CAD build for the part. Positions are in the model's coordinates, mm. Give positions to 0.01 mm unless a question says otherwise; leave off trailing zeros. Write each loop counter-clockwise with the first axis right and the second up, starting at its lowest first coordinate (ties: lowest second). Pieces come first, ordered by that corner, then holes. Notation, with made-up numbers: (51.5, 76) - (107.5, 76) arc R18 cw to (107.5, 97) - close; hole circle Ø8 at (29, 27). An arc over 180 degrees is marked (long way). Answer as a JSON object with one key per item and string values.
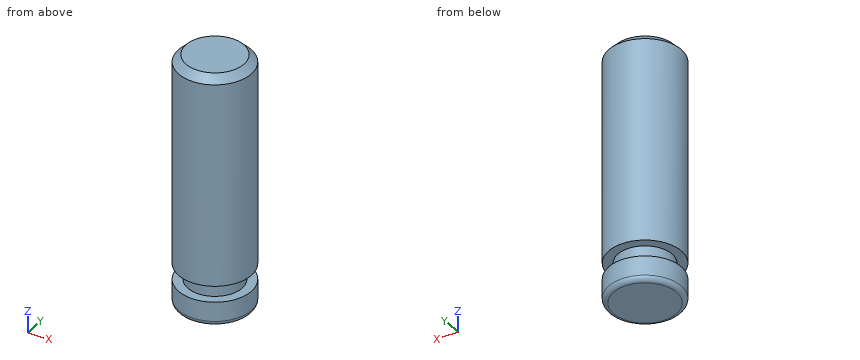
from build123d import *

# Parameters (mm, degrees)
SKETCH1_R      = 1.9558
EXTRUDE1_DEPTH = 6.7437
SKETCH2_W      = 0.4953
SKETCH2_H      = 0.8636
FILLET1_R      = 0.254
CHAMFER1_SIZE  = 0.396875


with BuildPart() as part:
    # Sketch1 → Extrude1 (new body, symmetric)
    with BuildSketch(Plane.XY):
        Circle(SKETCH1_R)
    extrude(amount=EXTRUDE1_DEPTH, both=True)

    # Sketch2 → Cut-Revolve1 (revolve, cut)
    with BuildSketch(Plane(origin=(0, 0, 0), x_dir=(1, 0, 0), z_dir=(0, 1, 0))):
        with Locations((1.70815, 5.0165)):
            Rectangle(SKETCH2_W, SKETCH2_H)
    revolve(axis=Axis((0, 0, -10.042474892), (0, 0, 1)), mode=Mode.SUBTRACT)

    # Fillet1
    fillet1_edges = [part.edges().sort_by_distance(p)[0] for p in [
        (-1.9558, 0, -6.7437),
    ]]
    fillet(fillet1_edges, radius=FILLET1_R)

    # Chamfer1
    chamfer1_edges = [part.edges().sort_by_distance(p)[0] for p in [
        (-1.9558, 0, 6.7437),
    ]]
    chamfer(chamfer1_edges, length=CHAMFER1_SIZE)


solid = part.part
Item 1: Cut at C-C (z = -2.5). Give the cut face in (x, y).
Entries:
{"outline": "circle Ø3.91 at (0, 0)"}
Item 2: Flat gauge pin, fed straight in: P1, Ø1.5, axis at x = -1.5, z = 0, coming from the +Y side. Where does the tip first touch, or does it go through?
Entries:
{"P1": "y = 1.81"}
Item 3: Probe line 1 (Z direction, x = -0.75, y = -1.3); line 2 (Z direction, x = 1.1, y = 1.45); line 3 (Y direction, x = -1.3, z = 3.5). List the from-to ranges inside material, lowest first. Write a range as from..to.
Entries:
{"line 1": "-6.74..-5.45, -4.58..6.74", "line 2": "-6.71..-5.45, -4.58..6.48", "line 3": "-1.46..1.46"}
Item 4: Cut at A-A (x = 0). Give the cut face in (y, z).
Entries:
{"outline": "(-1.96, -6.49) arc R0.25 ccw to (-1.7, -6.74) - (1.7, -6.74) arc R0.25 ccw to (1.96, -6.49) - (1.96, -5.45) - (1.46, -5.45) - (1.46, -4.58) - (1.96, -4.58) - (1.96, 6.35) - (1.56, 6.74) - (-1.56, 6.74) - (-1.96, 6.35) - (-1.96, -4.58) - (-1.46, -4.58) - (-1.46, -5.45) - (-1.96, -5.45) - close"}
